from build123d import *

# Parameters (mm, degrees)
SKETCH_1_W          = 120
SKETCH_1_H          = 100
EXTRUDE_1_DEPTH     = 4
FILLET_1_R          = 14
SKETCH_2_R          = 1.5
CUT_EXTRUDE_1_DEPTH = 5
SKETCH_7_R          = 2.5
CUT_EXTRUDE_2_DEPTH = 5


with BuildPart() as part:
    # 草图1 → 凸台-拉伸1 (new body)
    with BuildSketch(Plane.XY):
        with Locations((7.34439834, -11.161825726)):
            Rectangle(SKETCH_1_W, SKETCH_1_H)
    extrude(amount=EXTRUDE_1_DEPTH)

    # 圆角1
    fillet_1_edges = [part.edges().sort_by_distance(p)[0] for p in [
        (-52.65560166, 38.838174274, 2),
        (67.34439834, 38.838174274, 2),
        (67.34439834, -61.161825726, 2),
        (-52.65560166, -61.161825726, 2),
    ]]
    fillet(fillet_1_edges, radius=FILLET_1_R)

    # 草图2 → 切除-拉伸1 (cut, through all)
    with BuildSketch(Plane.XY.offset(4)):
        with Locations((53.34439834, 24.838174274)):
            Circle(SKETCH_2_R)
        with Locations((-38.65560166, 24.838174274)):
            Circle(SKETCH_2_R)
        with Locations((-38.65560166, -47.161825726)):
            Circle(SKETCH_2_R)
        with Locations((53.34439834, -47.161825726)):
            Circle(SKETCH_2_R)
    extrude(amount=-CUT_EXTRUDE_1_DEPTH, mode=Mode.SUBTRACT)

    # 草图7 → 切除-拉伸2 (cut, through all)
    with BuildSketch(Plane(origin=(0, 0, 0), x_dir=(-1, 0, 0), z_dir=(0, 0, -1))):
        with Locations((-44.84439834, -11.161825726)):
            Circle(SKETCH_7_R)
        with Locations((-29.84439834, -11.161825726)):
            Circle(SKETCH_7_R)
    extrude(amount=-CUT_EXTRUDE_2_DEPTH, mode=Mode.SUBTRACT)


solid = part.part
Design review of the part built by this model. Coordinates are the model's own, in mm. Coordinates: 2 decimals unless noted, no trailing zeros. Order: outer loops, then holes, each group sorted by start corner. A loop starts at its lowest first (then second) coordinate and runs counter-clockwise, first axis right, second up. Notation, with made-up numbers: (69, -31) - (82, -31) arc R32 ccw to (82, -3) - close; hole circle Ø6 at (87.25, 33). An arc over 180 degrees is marked (long way). Put each result on its own line as item: value.
1) Take a section at A-A, the plane z = 0.8. Give the boundary of the cut face in (x, y).
Response values:
outline: (-52.66, -47.16) arc R14 ccw to (-38.66, -61.16) - (53.34, -61.16) arc R14 ccw to (67.34, -47.16) - (67.34, 24.84) arc R14 ccw to (53.34, 38.84) - (-38.66, 38.84) arc R14 ccw to (-52.66, 24.84) - close; hole circle Ø3 at (-38.66, -47.16); hole circle Ø3 at (-38.66, 24.84); hole circle Ø5 at (29.84, -11.16); hole circle Ø5 at (44.84, -11.16); hole circle Ø3 at (53.34, -47.16); hole circle Ø3 at (53.34, 24.84)
2) The part is to be moulded in two halves that separate along X. For faces 1 (the face through (63.134, -57.17, 2.028)), 2 (the face through (7, -10, 4)), 3 (the face through (-48.66, 34.63, 2.03)), 4 (the face through (54.775, 25.289, 2.028)), say which applies: released by +X, released by -X, zero draft, split by the parting line, or undercut.
Response values:
face 1: released by +X
face 2: zero draft
face 3: released by -X
face 4: undercut
3) Wall thickness on L1, parallel to X at y = -10, z = 0.25; L2, parallel to Y at x = 47, z = 2.45; L3, parallel to X at y = -49.5, z = 0.2: over which ranges is each line inside the solid? List them lowest first. Write a range as from..to.
Response values:
L1: x = -52.66..27.63, 32.06..42.63, 47.06..67.34
L2: y = -61.16..-12.43, -9.9..38.84
L3: x = -52.46..67.15
